Part model, mm, in its own coordinate system. A direction names the side the tool comes from. Give positions to 0.01 mm unless a question says otherwise; leave off trailing zeros. Order: outer loops, then holes, each group sorted by start corner. A loop starts at its lowest first (then second) coordinate and runs counter-clockwise, first axis right, second up.
1. Slice it at B-B on x = 0. List the corners of the cut face in (y, z), and give its area (3 significant figures).
2. Drop flat-ended pins along their axis: pin 1 Ø5 at (y, z) = (-6.5, 3.5) entering from -X; pin 2 Ø4.5 at (y, z) = (-0.5, 12.5) entering from +X; pin 3 Ø2.5 at (y, z) = (-6.5, 3) entering from +X. Give the stop position or say it passes through.
3. Slice it at D-D on z = 5.5. List the corners of the cut face in (x, y), and give its area (3 significant figures).
4. Mould opens along Y. For faces 6 (the flat face through (6.59, -1.97, 2.35)), 7 (the flat face through (-1, 2.794, 17)), 8 (the cylindrical face through (4.804, 8.225, 2.348)), 9 (the cylindrical face through (3.175, -0.048, 16.647)) say: +Y half, -Y half, draft (parallel to the pull), parting line (faces both ways), or undercut.
5. Probe line 1 (X direction, y = 0.25, z = 1); line 2 (X direction, y = -4.25, z = 1); line 3 (Z direction, x = 0.75, y = 7.75). List the from-to ranges inside material, lowest first.
6. Which spindle directions (+Z, -Z, +X, -X, +Y, -Y) get a long thin tool onto all of the face, cutting with end or side? Do faces 1 (the flat face through (3, 0, 16.256)), 2 (the flat face through (-0.508, 0, 14)), 3 (the flat face through (-1, -2.794, 17)), 4 (the flat face through (0, -5, 4.762)), 5 (the flat face through (-6.527, -1.935, 2.348)). Say none if no direction does.
7. Slice it at A-A on y = 0. Give the number of separate pieces and of enclosed holes in the cut face, and give its area (3 significant figures).
from build123d import *

# Parameters (mm, degrees)
SKETCH1_R           = 4.233333333
BOSS_EXTRUDE1_DEPTH = 6.35
BOSS_EXTRUDE2_DEPTH = 4.7625
SKETCH1_4_R         = 12.7
SKETCH1_4_R_2       = 9.525
BOSS_EXTRUDE3_DEPTH = 4.7625
SKETCH2_R           = 2.794
BOSS_EXTRUDE4_DEPTH = 9.906
SKETCH3_R           = 3.175
BOSS_EXTRUDE5_DEPTH = 1.5875
SKETCH4_W           = 8.466666667
SKETCH4_H           = 6.35
CUT_EXTRUDE1_DEPTH  = 0.508
SKETCH5_W           = 6.35
SKETCH5_H           = 1.439333333
SKETCH5_W_2         = 8.466666666
CUT_EXTRUDE2_DEPTH  = 1.5875
CHAMFER1_SIZE       = 0.79375
CHAMFER1_SIZE2      = 0.458271776
CHAMFER2_SIZE       = 0.79375
CHAMFER2_SIZE2      = 0.458271776


with BuildPart() as part:
    # Sketch1 → Boss-Extrude1 (new body)
    with BuildSketch(Plane.XY):
        Circle(SKETCH1_R)
    extrude(amount=BOSS_EXTRUDE1_DEPTH)

    # Sketch1_3 → Boss-Extrude2 (add)
    with BuildSketch(Plane.XY):
        with BuildLine():
            Line((7.33976717, 6.070703656), (2.604884453, 3.337017845))
            ThreePointArc((2.604884453, 3.337017845), (3.666174209, 2.116666667), (4.192384453, 0.587387188))
            Line((4.192384453, 0.587387188), (8.92726717, 3.321072999))
            ThreePointArc((8.92726717, 3.321072999), (8.248891971, 4.7625), (7.33976717, 6.070703656))
        make_face()
        with BuildLine():
            Line((8.92726717, -3.321072999), (4.192384453, -0.587387188))
            ThreePointArc((4.192384453, -0.587387188), (3.666174209, -2.116666667), (2.604884453, -3.337017845))
            Line((2.604884453, -3.337017845), (7.33976717, -6.070703656))
            ThreePointArc((7.33976717, -6.070703656), (8.248891971, -4.7625), (8.92726717, -3.321072999))
        make_face()
        with BuildLine():
            ThreePointArc((1.5875, -3.924405033), (0, -4.233333333), (-1.5875, -3.924405033))
            Line((-1.5875, -3.924405033), (-1.5875, -9.391776656))
            ThreePointArc((-1.5875, -9.391776656), (0, -9.525), (1.5875, -9.391776656))
            Line((1.5875, -9.391776656), (1.5875, -3.924405033))
        make_face()
        with BuildLine():
            ThreePointArc((-2.604884453, -3.337017845), (-3.666174209, -2.116666667), (-4.192384453, -0.587387188))
            Line((-4.192384453, -0.587387188), (-8.92726717, -3.321072999))
            ThreePointArc((-8.92726717, -3.321072999), (-8.248891971, -4.7625), (-7.33976717, -6.070703656))
            Line((-7.33976717, -6.070703656), (-2.604884453, -3.337017845))
        make_face()
        with BuildLine():
            ThreePointArc((-4.192384453, 0.587387188), (-3.666174209, 2.116666667), (-2.604884453, 3.337017845))
            Line((-2.604884453, 3.337017845), (-7.33976717, 6.070703656))
            ThreePointArc((-7.33976717, 6.070703656), (-8.248891971, 4.7625), (-8.92726717, 3.321072999))
            Line((-8.92726717, 3.321072999), (-4.192384453, 0.587387188))
        make_face()
        with BuildLine():
            Line((-1.5875, 9.391776656), (-1.5875, 3.924405033))
            ThreePointArc((-1.5875, 3.924405033), (0, 4.233333333), (1.5875, 3.924405033))
            Line((1.5875, 3.924405033), (1.5875, 9.391776656))
            ThreePointArc((1.5875, 9.391776656), (0, 9.525), (-1.5875, 9.391776656))
        make_face()
    extrude(amount=BOSS_EXTRUDE2_DEPTH)

    # Sketch1_4 → Boss-Extrude3 (add)
    with BuildSketch(Plane.XY):
        Circle(SKETCH1_4_R)
        Circle(SKETCH1_4_R_2, mode=Mode.SUBTRACT)
    extrude(amount=BOSS_EXTRUDE3_DEPTH)

    # Sketch2 → Boss-Extrude4 (add)
    with BuildSketch(Plane.XY.offset(6.35)):
        Circle(SKETCH2_R)
    extrude(amount=BOSS_EXTRUDE4_DEPTH)

    # Sketch3 → Boss-Extrude5 (add)
    with BuildSketch(Plane.XY.offset(16.256)):
        Circle(SKETCH3_R)
    extrude(amount=BOSS_EXTRUDE5_DEPTH)

    # Sketch4 → Cut-Extrude1 (cut, symmetric)
    with BuildSketch(Plane(origin=(0, 0, 0), x_dir=(0, 0, -1), z_dir=(1, 0, 0))):
        with Locations((-13.610166667, 0)):
            Rectangle(SKETCH4_W, SKETCH4_H)
    extrude(amount=CUT_EXTRUDE1_DEPTH, both=True, mode=Mode.SUBTRACT)

    # Sketch5 → Cut-Extrude2 (cut)
    with BuildSketch(Plane.XY.offset(17.8435)):
        with Locations((0, 3.513666666)):
            Rectangle(SKETCH5_W, SKETCH5_H)
        with Locations((0, -3.513666666)):
            Rectangle(SKETCH5_W_2, SKETCH5_H)
    extrude(amount=-CUT_EXTRUDE2_DEPTH, mode=Mode.SUBTRACT)

    # Chamfer1
    chamfer1_edges = [part.edges().sort_by_distance(p)[0] for p in [
        (-3.175, 0, 17.8435),
    ]]
    chamfer1_side = [part.faces().sort_by_distance(p)[0] for p in [
        (-3.175, 0, 17.04975),
    ]]
    chamfer(chamfer1_edges, length=CHAMFER1_SIZE, length2=CHAMFER1_SIZE2, reference=chamfer1_side[0])

    # Chamfer2
    chamfer2_edges = [part.edges().sort_by_distance(p)[0] for p in [
        (3.175, 0, 17.8435),
    ]]
    chamfer2_side = [part.faces().sort_by_distance(p)[0] for p in [
        (3.175, 0, 17.04975),
    ]]
    chamfer(chamfer2_edges, length=CHAMFER2_SIZE, length2=CHAMFER2_SIZE2, reference=chamfer2_side[0])


solid = part.part
Data:
1. outline: (-12.7, 0) - (12.7, 0) - (12.7, 4.76) - (4.23, 4.76) - (4.23, 6.35) - (2.79, 6.35) - (2.79, 9.38) - (-2.79, 9.38) - (-2.79, 6.35) - (-4.23, 6.35) - (-4.23, 4.76) - (-12.7, 4.76) - close
1. area: 151 mm2
2. pin 1: stops at x = -12.05
2. pin 2: stops at x = 2.79
2. pin 3: stops at x = 11.56
3. outline: circle Ø8.47 at (0, 0)
3. area: 56.3 mm2
4. face 6: undercut
4. face 7: +Y half
4. face 8: undercut
4. face 9: parting line
5. line 1: x = -12.7 to -9.52, -4.23 to 4.23, 9.52 to 12.7
5. line 2: x = -11.97 to -4.19, -1.59 to 1.59, 4.19 to 11.97
5. line 3: z = 0 to 4.76
6. face 1: +X
6. face 2: +Z, +Y, -Y
6. face 3: +Z, +X, -X, -Y
6. face 4: +Z
6. face 5: +Z, -Z
7. separate pieces: 3
7. enclosed holes: 0
7. area: 140 mm2
